Design review of the part built by this model. Coordinates are the model's own, in mm. Face numbers are marked on the shaded views. Round coordinates to 2 decimals unless told otherwise and drop trailing zeros. Order: outer loops, then holes, each group sorted by start corner. A loop starts at its lowest first (then second) coordinate and runs counter-clockwise, first axis right, second up. Notation, with made-up numbers: (-20.75, 20.5) - (15.25, 20.5) arc R9 ccw to (15.25, 35.5) - close; hole circle Ø3 at (72, 3.5). An arc over 180 degrees is marked (long way). Write item = value, one per line.
from build123d import *

# Parameters (mm, degrees)
F0_R     = 10
F1_DEPTH = 5
F2_R     = 5
F3_R     = 5
F4_DEPTH = 25


with BuildPart() as f1:
    # F0 (on Front) → F1 (new body)
    with BuildSketch(Plane.XZ):
        with BuildLine():
            add(Edge.make_bspline(
                [(19.6117025062, -3.4953018185), (20.0776619455, -2.3335824214), (20.6438929209, -0.0613566909), (20.1493664179, 2.2303480995), (19.742406118, 3.3519886549)],
                knots=[0.4195745688, 0.4195745688, 0.4195745688, 0.4195745688, 0.4960722568, 0.5688744263, 0.5688744263, 0.5688744263, 0.5688744263], degree=3))
            Line((19.742406118, 3.3519886549), (14.6206761833, 3.3519886549))
            ThreePointArc((14.6206761833, 3.3519886549), (14.9048673719, 1.6866916212), (15, 0))
            ThreePointArc((15, 0), (14.8964119942, -1.7598038809), (14.5870787068, -3.4953018185))
            Line((14.5870787068, -3.4953018185), (19.6117025062, -3.4953018185))
        make_face()
        with BuildLine():
            add(Edge.make_bspline(
                [(-1.5163984723, -18.1465453552), (-0.9012756584, -17.6861315251), (-0.0133596841, -17.0968852874), (0.8972354155, -17.4862781525), (1.5163984723, -17.845237755)],
                knots=[0.3644446734, 0.3644446734, 0.3644446734, 0.3644446734, 0.5028904355, 0.6389885865, 0.6389885865, 0.6389885865, 0.6389885865], degree=3))
            Line((1.5163984723, -17.845237755), (1.5163984723, -14.9231543473))
            ThreePointArc((1.5163984723, -14.9231543473), (0, -15), (-1.5163984723, -14.9231543473))
            Line((-1.5163984723, -14.9231543473), (-1.5163984723, -18.1465453552))
        make_face()
        with BuildLine():
            Line((-14.6757838937, 3.1018328621), (-19.1463490467, 3.1018328621))
            add(Edge.make_bspline(
                [(-19.1463490467, 3.1018328621), (-19.4804537552, 2.0677531569), (-19.877871021, 0), (-19.4804537552, -2.0677531569), (-19.1463490467, -3.1018328621)],
                knots=[0.434082988, 0.434082988, 0.434082988, 0.434082988, 0.5, 0.565917012, 0.565917012, 0.565917012, 0.565917012], degree=3))
            Line((-19.1463490467, -3.1018328621), (-14.6757838937, -3.1018328621))
            ThreePointArc((-14.6757838937, -3.1018328621), (-15, 0), (-14.6757838937, 3.1018328621))
        make_face()
        with BuildLine():
            Line((1.225561158, 14.9498494925), (1.225561158, 17.9168751217))
            add(Edge.make_bspline(
                [(1.225561158, 17.9168751217), (0.7517359921, 17.6368227378), (0, 17.3228835959), (-0.7517359921, 17.6368227378), (-1.225561158, 17.9168751217)],
                knots=[0.3852289018, 0.3852289018, 0.3852289018, 0.3852289018, 0.5, 0.6147710982, 0.6147710982, 0.6147710982, 0.6147710982], degree=3))
            Line((-1.225561158, 17.9168751217), (-1.225561158, 14.9498494925))
            ThreePointArc((-1.225561158, 14.9498494925), (0, 15), (1.225561158, 14.9498494925))
        make_face()
        with BuildLine():
            Line((27.5, -12.5), (27.5, 12.5))
            ThreePointArc((27.5, 12.5), (18.3695172954, 15.5989796412), (13.0117252596, 23.6154285891))
            add(Edge.make_bspline(
                [(19.742406118, 3.3519886549), (17.3324368296, 9.9942072978), (9.1074771998, 16.7819842724), (13.0117252596, 23.6154285891)],
                knots=[0.5688744263, 0.5688744263, 0.5688744263, 0.5688744263, 1, 1, 1, 1], degree=3))
            add(Edge.make_bspline(
                [(19.6117025062, -3.4953018185), (20.0776619455, -2.3335824214), (20.6438929209, -0.0613566909), (20.1493664179, 2.2303480995), (19.742406118, 3.3519886549)],
                knots=[0.4195745688, 0.4195745688, 0.4195745688, 0.4195745688, 0.4960722568, 0.5688744263, 0.5688744263, 0.5688744263, 0.5688744263], degree=3))
            add(Edge.make_bspline(
                [(13.0117252596, -22.8125530654), (9.2106265425, -16.1632445639), (17.0560078684, -9.8671011282), (19.6117025062, -3.4953018185)],
                knots=[0, 0, 0, 0, 0.4195745688, 0.4195745688, 0.4195745688, 0.4195745688], degree=3))
            add(Edge.make_bspline(
                [(1.5163984723, -17.845237755), (3.1587788316, -18.7974072918), (5.9815411198, -20.9170774405), (13.0117252596, -22.8125530654)],
                knots=[0.6389885865, 0.6389885865, 0.6389885865, 0.6389885865, 1, 1, 1, 1], degree=3))
            add(Edge.make_bspline(
                [(-1.5163984723, -18.1465453552), (-0.9012756584, -17.6861315251), (-0.0133596841, -17.0968852874), (0.8972354155, -17.4862781525), (1.5163984723, -17.845237755)],
                knots=[0.3644446734, 0.3644446734, 0.3644446734, 0.3644446734, 0.5028904355, 0.6389885865, 0.6389885865, 0.6389885865, 0.6389885865], degree=3))
            add(Edge.make_bspline(
                [(-13.0117252596, -23.6154285891), (-5.9146832629, -21.7019267737), (-3.1356479862, -19.3585388852), (-1.5163984723, -18.1465453552)],
                knots=[0, 0, 0, 0, 0.3644446734, 0.3644446734, 0.3644446734, 0.3644446734], degree=3))
            ThreePointArc((-13.0117252596, -23.6154285891), (-12.6284815653, -25.5409340371), (-12.5, -27.5))
            Line((-12.5, -27.5), (12.5, -27.5))
            ThreePointArc((12.5, -27.5), (16.8933982822, -16.8933982822), (27.5, -12.5))
        make_face()
        with BuildLine():
            ThreePointArc((-13.0117252596, 23.6154285891), (-18.3695172954, 15.5989796412), (-27.5, 12.5))
            Line((-27.5, 12.5), (-27.5, -12.5))
            ThreePointArc((-27.5, -12.5), (-18.3695172954, -15.5989796412), (-13.0117252596, -23.6154285891))
            add(Edge.make_bspline(
                [(-19.1463490467, -3.1018328621), (-16.9461708863, -9.9115530651), (-8.8743910836, -16.7300820857), (-13.0117252596, -23.6154285891)],
                knots=[0.565917012, 0.565917012, 0.565917012, 0.565917012, 1, 1, 1, 1], degree=3))
            add(Edge.make_bspline(
                [(-19.1463490467, 3.1018328621), (-19.4804537552, 2.0677531569), (-19.877871021, 0), (-19.4804537552, -2.0677531569), (-19.1463490467, -3.1018328621)],
                knots=[0.434082988, 0.434082988, 0.434082988, 0.434082988, 0.5, 0.565917012, 0.565917012, 0.565917012, 0.565917012], degree=3))
            add(Edge.make_bspline(
                [(-13.0117252596, 23.6154285891), (-8.8743910836, 16.7300820857), (-16.9461708863, 9.9115530651), (-19.1463490467, 3.1018328621)],
                knots=[0, 0, 0, 0, 0.434082988, 0.434082988, 0.434082988, 0.434082988], degree=3))
        make_face()
        with BuildLine():
            ThreePointArc((13.0117252596, 23.6154285891), (12.6284815653, 25.5409340371), (12.5, 27.5))
            Line((12.5, 27.5), (-12.5, 27.5))
            ThreePointArc((-12.5, 27.5), (-12.6284815653, 25.5409340371), (-13.0117252596, 23.6154285891))
            add(Edge.make_bspline(
                [(-1.225561158, 17.9168751217), (-2.8159541317, 18.856870242), (-5.5099399576, 21.1835256037), (-13.0117252596, 23.6154285891)],
                knots=[0.6147710982, 0.6147710982, 0.6147710982, 0.6147710982, 1, 1, 1, 1], degree=3))
            add(Edge.make_bspline(
                [(1.225561158, 17.9168751217), (0.7517359921, 17.6368227378), (0, 17.3228835959), (-0.7517359921, 17.6368227378), (-1.225561158, 17.9168751217)],
                knots=[0.3852289018, 0.3852289018, 0.3852289018, 0.3852289018, 0.5, 0.6147710982, 0.6147710982, 0.6147710982, 0.6147710982], degree=3))
            add(Edge.make_bspline(
                [(13.0117252596, 23.6154285891), (5.5099399576, 21.1835256037), (2.8159541317, 18.856870242), (1.225561158, 17.9168751217)],
                knots=[0, 0, 0, 0, 0.3852289018, 0.3852289018, 0.3852289018, 0.3852289018], degree=3))
        make_face()
        with BuildLine():
            ThreePointArc((27.5, 12.5), (38.1066017178, 16.8933982822), (42.5, 27.5))
            ThreePointArc((42.5, 27.5), (27.5, 42.5), (12.5, 27.5))
            ThreePointArc((12.5, 27.5), (12.6284815653, 25.5409340371), (13.0117252596, 23.6154285891))
            ThreePointArc((13.0117252596, 23.6154285891), (18.3695172954, 15.5989796412), (27.5, 12.5))
        make_face()
        with Locations((27.5, 27.5)):
            Circle(F0_R, mode=Mode.SUBTRACT)
        with BuildLine():
            ThreePointArc((15, 0), (14.9048673719, 1.6866916212), (14.6206761833, 3.3519886549))
            ThreePointArc((14.6206761833, 3.3519886549), (9.8185234873, 11.3400439386), (1.225561158, 14.9498494925))
            ThreePointArc((1.225561158, 14.9498494925), (0, 15), (-1.225561158, 14.9498494925))
            ThreePointArc((-1.225561158, 14.9498494925), (-9.9149920894, 11.2557954791), (-14.6757838937, 3.1018328621))
            ThreePointArc((-14.6757838937, 3.1018328621), (-15, 0), (-14.6757838937, -3.1018328621))
            ThreePointArc((-14.6757838937, -3.1018328621), (-10.0241010997, -11.1587363596), (-1.5163984723, -14.9231543473))
            ThreePointArc((-1.5163984723, -14.9231543473), (0, -15), (1.5163984723, -14.9231543473))
            ThreePointArc((1.5163984723, -14.9231543473), (9.8731680665, -11.2924998265), (14.5870787068, -3.4953018185))
            ThreePointArc((14.5870787068, -3.4953018185), (14.8964119942, -1.7598038809), (15, 0))
        make_face()
        Circle(F0_R, mode=Mode.SUBTRACT)
        with BuildLine():
            ThreePointArc((42.5, -27.5), (38.1066017178, -16.8933982822), (27.5, -12.5))
            ThreePointArc((27.5, -12.5), (16.8933982822, -16.8933982822), (12.5, -27.5))
            ThreePointArc((12.5, -27.5), (27.5, -42.5), (42.5, -27.5))
        make_face()
        with Locations((27.5, -27.5)):
            Circle(F0_R, mode=Mode.SUBTRACT)
        with BuildLine():
            ThreePointArc((-13.0117252596, -23.6154285891), (-18.3695172954, -15.5989796412), (-27.5, -12.5))
            ThreePointArc((-27.5, -12.5), (-38.1066017178, -38.1066017178), (-12.5, -27.5))
            ThreePointArc((-12.5, -27.5), (-12.6284815653, -25.5409340371), (-13.0117252596, -23.6154285891))
        make_face()
        with Locations((-27.5, -27.5)):
            Circle(F0_R, mode=Mode.SUBTRACT)
        with BuildLine():
            ThreePointArc((-13.0117252596, 23.6154285891), (-12.6284815653, 25.5409340371), (-12.5, 27.5))
            ThreePointArc((-12.5, 27.5), (-38.1066017178, 38.1066017178), (-27.5, 12.5))
            ThreePointArc((-27.5, 12.5), (-18.3695172954, 15.5989796412), (-13.0117252596, 23.6154285891))
        make_face()
        with Locations((-27.5, 27.5)):
            Circle(F0_R, mode=Mode.SUBTRACT)
    extrude(amount=F1_DEPTH)

    # F2
    f2_edges = [f1.edges().sort_by_distance(p)[0] for p in [
        (27.5, -2.5, -12.5),
    ]]
    fillet(f2_edges, radius=F2_R)

    # F3
    f3_edges = [f1.edges().sort_by_distance(p)[0] for p in [
        (-27.5, -2.5, -12.5),
        (-12.5, -2.5, 27.5),
        (27.5, -2.5, 12.5),
    ]]
    fillet(f3_edges, radius=F3_R)


with BuildPart() as f4:
    # F0 (on Front) → F4 (new body)
    with BuildSketch(Plane.XZ):
        Circle(F0_R)
    extrude(amount=F4_DEPTH)


solid = f1.part
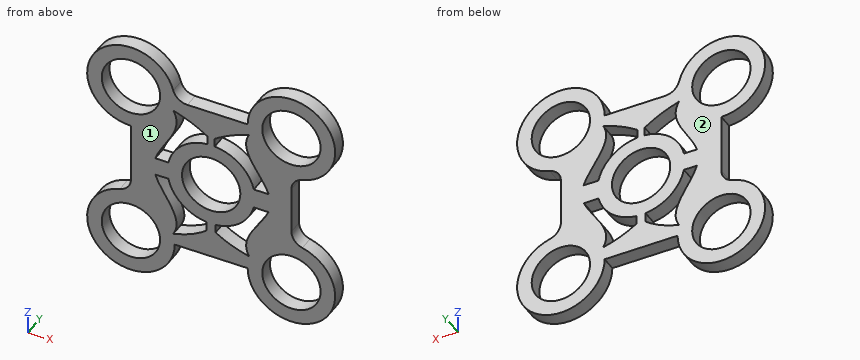
1) We need section D-D on y = -3.1. Give the number of separate pieces and of enclosed holes in the cut face, and give its area (3 significant figures).
Findings:
separate_pieces = 1
enclosed_holes = 9
area = 3,080 mm^2
2) We need section A-A on z = 0. Write out the cut boundary in (x, y).
Findings:
outline = (-27.5, -5) - (-10, -5) - (-10, 0) - (-27.5, 0) - close; (10, -5) - (27.5, -5) - (27.5, 0) - (10, 0) - close
3) Clearance check with flat-ended pins moving along their axes: pin 1 Ø1 at (y, z) = (-1.5, 6) entering from +X; pin 2 Ø1.5 at (x, y) = (4.5, -3) entering from +Z; pin 3 Ø1.5 at (x, y) = (5, -3.5) entering from -Z; pin 4 Ø12 at (x, z) = (-27.5, 27.5) entering from +Y. State where each tip first meets the part, or that it passes through.
Findings:
pin_1 = 27.5
pin_2 = 27.5
pin_3 = -27.5
pin_4 = through
4) The part is to be moulded in two halves that separate along Y. For the marked faces 1 and 2, say which applies: released by +Y, released by -Y, zero draft, split by the parting line, or undercut.
Findings:
face_1 = released by -Y
face_2 = released by +Y
5) We need section C-C on x = -25. Write out the cut boundary in (y, z).
Findings:
outline = (-5, -42.29) - (0, -42.29) - (0, -37.18) - (-5, -37.18) - close; (-5, -17.82) - (0, -17.82) - (0, 17.82) - (-5, 17.82) - close; (-5, 37.18) - (0, 37.18) - (0, 42.29) - (-5, 42.29) - close
6) We need section B-B on x = 0. Write out the cut boundary in (y, z), and give its area (3 significant figures).
Findings:
outline = (-5, -27.5) - (0, -27.5) - (0, -10) - (-5, -10) - close; (-5, 10) - (0, 10) - (0, 27.5) - (-5, 27.5) - close
area = 175 mm^2
7) To check wall thickness, follow L1, parallel to Z at x = 23.5, y = -1.5; L2, parallel to X at y = -3.25, z = -9; L3, parallel to Z at x = 0, y = -1.25. State the ranges of each line that lie inside material, in increasing order. Write a range as from..to.
Findings:
L1 = -41.96..-36.67, -18.33..18.33, 36.67..41.96
L2 = -27.58..-16.21, -12..-4.36, 4.36..12, 16.49..27.58
L3 = -27.5..-10, 10..27.5
